Part print with two shaded views. Sizes in mm from the minimum x, y, z corner. A direction names the side the tool comes from. Round coordinates to 2 decimals unless told otherwise and drop trailing zeros. Loops run counter-clockwise (first coordinate to the right, second up) from the corner with the lowest first, then second, coordinate; pieces in that order, holes last. Notation, with made-up numbers: M -38.75,7 L -34.75,7 A20 cw -34.75,17 Z; hole C -27,18.5 d5. An arc over 180 degrees is marked long. Use a Markdown table: item, result. Add a question column.
Item 1: Pin check, flat tips, straight feed: P1, Ø6, axis at x = 8.5, z = 10.5, coming from the +Y side; P2, Ø4, axis at y = 21.5, z = 7.5, coming from the +X side; P3, Ø1.5, axis at y = 19.5, z = 6.5, coming from the +X side. Stop position of each tip, or through.
Item 2: Two-plate mould, pull along Y, no slides. Class the marked faces 5, 6, 7 and 8: +Y half, -Y half, draft (parallel to the pull), parting line (faces both ways), or undercut.
Item 3: Saw through at D-D on y = 6. Write the cut outline in (x, z).
Item 4: Saw through at A-A on z = 6. Give the number of separate pieces and of enclosed holes in the cut face, then the cut area to 3 significant figures.
Item 5: Saw through at B-B on x = 7. Write the cut outline in (y, z) (1 decimal).
Item 6: Wall check: L1, parallel to X at y = 4.25, z = 7.5; L2, parallel to Z at x = 7, y = 2.25; L3, parallel to Y at x = 30, z = 9.75. Give the ranges that are in metal, low to high. Write a range as from..to.
Item 7: Tool access for the marked faces 1, 2, 3 and 4: list every direction of +Z, -Z, +X, -X, +Y, -Y with a clear straight run to the whole face (end or side of a thin tool).
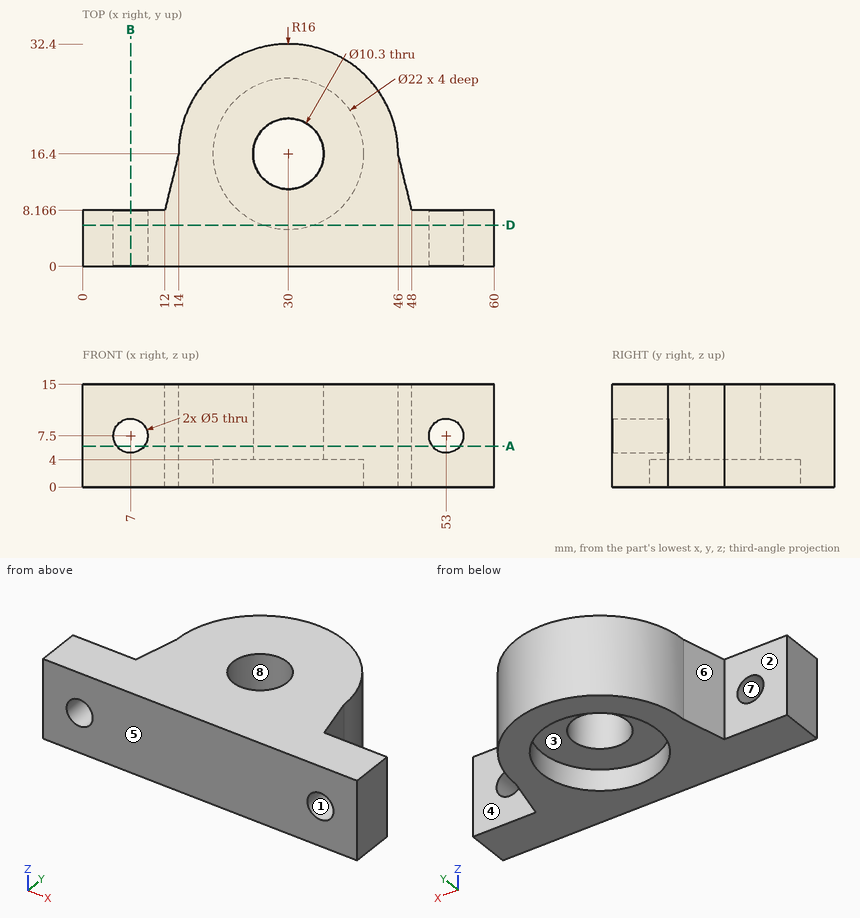
Entries:
| question | item | result |
|---|---|---|
| 1 | P1 | y = 8.17 |
| 1 | P2 | x = 45.7 |
| 1 | P3 | x = 45.83 |
| 2 | face 5 | -Y half |
| 2 | face 6 | +Y half |
| 2 | face 7 | draft |
| 2 | face 8 | undercut |
| 3 | outline | M 0,0 L 26.42,0 L 26.42,4 L 33.58,4 L 33.58,0 L 60,0 L 60,15 L 0,15 Z; hole C 7,7.5 d5; hole C 53,7.5 d5 |
| 4 | separate pieces | 3 |
| 4 | enclosed holes | 1 |
| 4 | area | 1,020 mm2 |
| 5 | outline | M 0,0 L 8.2,0 L 8.2,5 L 0,5 Z; M 0,10 L 8.2,10 L 8.2,15 L 0,15 Z |
| 6 | L1 | 0..4.5, 9.5..50.5, 55.5..60 |
| 6 | L2 | 0..5, 10..15 |
| 6 | L3 | 0..11.25, 21.55..32.4 |
| 7 | face 1 | +Y, -Y |
| 7 | face 2 | +Z, -Z, -X, +Y |
| 7 | face 3 | -Z |
| 7 | face 4 | +Z, -Z, +X, +Y |
